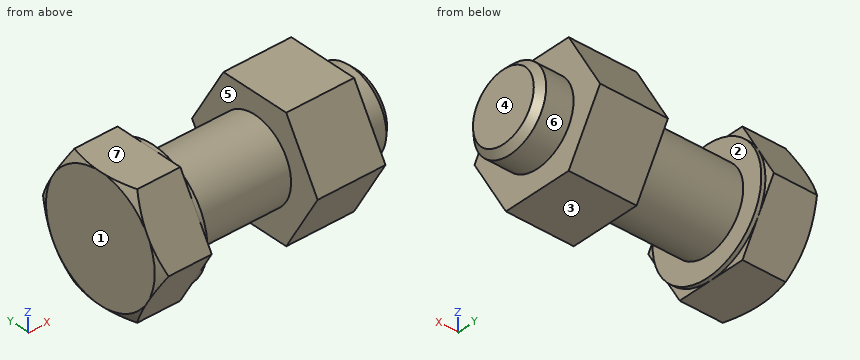
from build123d import *

# Parameters (mm, degrees)
BASEHEAD_DEPTH      = 7.76
SKETCH4_W           = 0.6
SKETCH4_H           = 11.392304845
BOSS_EXTRUDE1_DEPTH = 10


# Read off the part's stored shape, not the designer's step: HeadChamfer
with BuildPart() as part:
    # Sketch1 → BaseHead (new body)
    with BuildSketch(Plane(origin=(0, 0, 0), x_dir=(0, 0, -1), z_dir=(1, 0, 0))):
        Polygon((9, 5.196152423), (9, -5.196152423), (0, -10.392304845), (-9, -5.196152423), (-9, 5.196152423), (0, 10.392304845), align=None)
    extrude(amount=BASEHEAD_DEPTH)

    # HeadChamfer outline → HeadChamfer (revolve, cut)
    with BuildSketch(Plane.YX):
        Polygon((10.392304847, 0.803847578), (9, 0), (10.392304847, 0), align=None)
    revolve(axis=Axis((0, 0, 0), (1, 0, 0)), mode=Mode.SUBTRACT)

    # HeadChamfer 2 outline → HeadChamfer 2 (revolve)
    with BuildSketch(Plane.YX):
        Polygon((6, 7.76), (6, 36.796), (5.036, 37.76), (0, 37.76), (0, 7.76), align=None)
    revolve(axis=Axis((0, 0, 0), (1, 0, 0)))

    # Sketch4 → BearingFace (revolve, cut)
    with BuildSketch(Plane.XY, mode=Mode.PRIVATE) as bearingface_sk:
        with Locations((7.46, 14.696152423)):
            Rectangle(SKETCH4_W, SKETCH4_H)
    revolve(bearingface_sk.sketch.rotate(Axis((0, 0, 0), (1, 0, 0)), 90), axis=Axis((0, 0, 0), (1, 0, 0)), mode=Mode.SUBTRACT)

    # Sketch5 → Boss-Extrude1 (add)
    with BuildSketch(Plane(origin=(32.76, 0, 0), x_dir=(0, 0, -1), z_dir=(1, 0, 0))):
        Polygon((0, 10.392304845), (-9, 5.196152423), (-9, -5.196152423), (0, -10.392304845), (9, -5.196152423), (9, 5.196152423), align=None)
    extrude(amount=-BOSS_EXTRUDE1_DEPTH)


solid = part.part
Could you check a few things on this model? Use its own coordinates, in mm. Face numbers are marked on the shaded views. A direction names the side the tool comes from. Round coordinates to 2 decimals unless told otherwise and drop trailing zeros. Write each loop counter-clockwise with the first axis right and the second up, starting at its lowest first coordinate (ties: lowest second). Pieces come first, ordered by that corner, then holes. Notation, with made-up numbers: (54, -33) - (85, -33) arc R25 ccw to (85, -18) - close; hole circle Ø10 at (38.25, 89). An arc over 180 degrees is marked (long way). Put each result on its own line as item: value. Start each with the question number.
(1) Thinking about a two-plate mould opening in X: for the marked faces 1, 2, 3 and 4, which applies, released by +X, released by -X, zero draft, split by the parting line, or undercut?
(2) Will these pins go through, and if not, where does the flat tip stop? pin 1 (3 mm diameter, centred on y = 9.5, z = -1, fed in from +X); pin 2 (2 mm diameter, centred on x = 12.5, y = -3, fed in from -Z); pin 3 (9 mm diameter, centred on y = -2.5, z = 3, fed in from -X); pin 4 (5 mm diameter, centred on x = 17, y = -4, fed in from -Z).
(3) For the marked faces 5, 6 and 7, which set-ups out of +Z, -Z, +X, -X, +Y, -Y let a thin tool reach every point of the face, with its end or its side?
(4) I need wall thicknesses on probe 1 along X at (y, z) = (6.75, 3); probe 2 along X at (y, z) = (-5.5, -7.75); probe 3 along X at (y, z) = (-5.5, -2). Which ranges of each line are inside material? Lowest first, please.
(5) I want a section at A-A, the plane x = 17. Please give me the cut outline in (y, z), plus the area to 3 significant figures.
Here are the results:
1. face 1: released by -X
1. face 2: undercut
1. face 3: zero draft
1. face 4: released by +X
2. pin 1: stops at x = 32.76
2. pin 2: stops at z = -5.66
2. pin 3: stops at x = 0
2. pin 4: stops at z = -5.81
3. face 5: none
3. face 6: +X
3. face 7: +Z, +X, -X, +Y, -Y
4. probe 1: x = 0 to 7.76, 22.76 to 32.76
4. probe 2: x = 0.29 to 7.16, 22.76 to 32.76
4. probe 3: x = 0 to 36.94
5. outline: circle Ø12 at (0, 0)
5. area: 113 mm^2
